```python
from build123d import *

# Parameters (mm, degrees)
CROQUIS1_W                 = 19.8
CROQUIS1_H                 = 11.5
SALIENTE_EXTRUIR1_DEPTH    = 70.5
VACIADO1_T                 = -2
CROQUIS5_W                 = 15.8
CROQUIS5_H                 = 2
SALIENTE_EXTRUIR2_DEPTH    = 2
CROQUIS6_W                 = 19.8
CROQUIS6_H                 = 8
SALIENTE_EXTRUIR4_DEPTH    = 16
SALIENTE_EXTRUIR5_DEPTH    = 19.8
CROQUIS10_R                = 3
CORTAR_EXTRUIR4_DEPTH      = 19.8
CORTAR_EXTRUIR3_DEPTH      = 43.653516854
CORTAR_EXTRUIR3_DEPTH_BACK = 43.653516854
CROQUIS8_R                 = 1
CROQUIS11_W                = 15.8
CROQUIS11_H                = 26
CORTAR_EXTRUIR5_DEPTH      = 2
REDONDEO2_R                = 8
REDONDEO4_R                = 1
REDONDEO5_R                = 1
REDONDEO6_R                = 1
REDONDEO7_R                = 1
REDONDEO8_R                = 1


# Some blends are built 0.0001 mm under size
with BuildPart() as part:
    # Croquis1 → Saliente-Extruir1 (new body)
    with BuildSketch(Plane(origin=(0, 0, 0), x_dir=(0, 1, 0), z_dir=(0, 0, 1))):
        Rectangle(CROQUIS1_W, CROQUIS1_H)
    extrude(amount=SALIENTE_EXTRUIR1_DEPTH)

    # Vaciado1
    vaciado1_openings = [part.faces().sort_by_distance(p)[0] for p in [
        (0, 0, 70.5),
    ]]
    offset(amount=VACIADO1_T, openings=vaciado1_openings, kind=Kind.INTERSECTION)

    # Croquis5 → Saliente-Extruir2 (add)
    with BuildSketch(Plane.YZ.offset(5.75)):
        with Locations((0, 69.5)):
            Rectangle(CROQUIS5_W, CROQUIS5_H)
    extrude(amount=-SALIENTE_EXTRUIR2_DEPTH)

    # Croquis6 → Saliente-Extruir4 (add)
    with BuildSketch(Plane(origin=(-5.75, 0, 0), x_dir=(0, -1, 0), z_dir=(-1, 0, 0))):
        with Locations((0, 29)):
            Rectangle(CROQUIS6_W, CROQUIS6_H)
    extrude(amount=SALIENTE_EXTRUIR4_DEPTH)

    # Croquis9 → Saliente-Extruir5 (add)
    with BuildSketch(Plane.XZ.offset(9.9)):
        Polygon((-5.75, 70.5), (-12.75, 33), (-5.75, 33), align=None)
        Polygon((-5.75, 0), (-12.75, 25), (-5.75, 25), align=None)
    extrude(amount=-SALIENTE_EXTRUIR5_DEPTH)

    # Croquis10 → Cortar-Extruir4 (cut)
    with BuildSketch(Plane.XZ.offset(9.9)):
        with Locations(Location((-16.745253682, 29, 0), (0, 0, 270))):
            Circle(CROQUIS10_R)
    extrude(amount=-CORTAR_EXTRUIR4_DEPTH, mode=Mode.SUBTRACT)

    # Croquis8 → Cortar-Extruir3 (cut, two sides: drawn at the far end of the back side and taken through both)
    with BuildSketch(Plane(origin=(-4, 0, 33), x_dir=(1, 0, 0), z_dir=(0, 0, 1)).offset(-CORTAR_EXTRUIR3_DEPTH_BACK)):
        with Locations((-12.75, 5.1)):
            Circle(CROQUIS8_R)
        with Locations((-12.75, -4.9)):
            Circle(CROQUIS8_R)
    extrude(amount=CORTAR_EXTRUIR3_DEPTH + CORTAR_EXTRUIR3_DEPTH_BACK, mode=Mode.SUBTRACT)

    # Croquis11 → Cortar-Extruir5 (cut)
    with BuildSketch(Plane.YZ.offset(5.75)):
        with Locations((0, 15)):
            Rectangle(CROQUIS11_W, CROQUIS11_H)
    extrude(amount=-CORTAR_EXTRUIR5_DEPTH, mode=Mode.SUBTRACT)

    # Redondeo2
    # the kernel refuses this fillet: 8 mm, written as the material it adds along each edge
    with BuildSketch(Plane(origin=(5.75, -7.9, 28), x_dir=(0, 1, 0), z_dir=(-1, 0, 0)), Plane(origin=(5.75, 7.9, 28), x_dir=(0, 0, -1), z_dir=(-1, 0, 0))) as redondeo2_piece_1:
        with BuildLine():
            CenterArc((REDONDEO2_R, REDONDEO2_R), REDONDEO2_R, 180, 90)
            Line((0, REDONDEO2_R), (0, 0))
            Line((0, 0), (REDONDEO2_R, 0))
        make_face()
    extrude(amount=2)

    # Redondeo4
    redondeo4_edges = [part.edges().sort_by_distance(p)[0] for p in [
        (-12.75, 0, 33),
    ]]
    fillet(redondeo4_edges, radius=REDONDEO4_R)

    # Redondeo5
    redondeo5_edges = [part.edges().sort_by_distance(p)[0] for p in [
        (5.75, 0, 70.5),
        (-5.75, 0, 70.5),
    ]]
    fillet(redondeo5_edges, radius=REDONDEO5_R)

    # Redondeo6
    redondeo6_edges = [part.edges().sort_by_distance(p)[0] for p in [
        (-12.941660805, -9.9, 33.230748054),
        (-12.941660805, 9.9, 33.230748054),
        (-9.25, 9.9, 51.75),
        (-9.25, -9.9, 51.75),
        (-0.084696812, 9.9, 70.5),
        (5.75, 9.9, 34.75),
        (5.457106781, 9.9, 70.207106781),
        (-5.558339195, 9.9, 70.269251946),
        (-0.084696812, -9.9, 70.5),
        (5.75, -9.9, 34.75),
        (5.457106781, -9.9, 70.207106781),
        (-5.558339195, -9.9, 70.269251946),
        (-17.665303188, 9.9, 33),
        (-17.665303188, -9.9, 33),
    ]]
    fillet(redondeo6_edges, radius=REDONDEO6_R - 0.0001)  # a hair under: the kernel refuses the full size

    # Redondeo7
    redondeo7_edges = [part.edges().sort_by_distance(p)[0] for p in [
        (-0.49995, 9.9, 0),
        (5.75, 0, 0),
        (-0.49995, -9.9, 0),
        (5.457136071, -9.607136071, 0),
        (5.457136071, 9.607136071, 0),
        (-21.75, 0, 25),
    ]]
    fillet(redondeo7_edges, radius=REDONDEO7_R - 0.0001)  # a hair under: the kernel refuses the full size

    # Redondeo8
    redondeo8_edges = [part.edges().sort_by_distance(p)[0] for p in [
        (-21.75, 9.9, 29),
        (-21.75, 0, 33),
        (-21.75, -9.607136071, 32.707136071),
        (-21.75, 9.607136071, 32.707136071),
        (-21.75, -9.9, 29),
        (-16.75005, -9.9, 25),
        (-21.457136071, -9.9, 25.292863929),
        (-16.75005, 9.9, 25),
        (-21.457136071, 9.9, 25.292863929),
    ]]
    fillet(redondeo8_edges, radius=REDONDEO8_R - 0.0001)  # a hair under: the kernel refuses the full size


solid = part.part
```
Work out the finished part from the listing and answer in its coordinate system (mm). A direction names the side the tool comes from. Coordinates: 2 decimals unless noted, no trailing zeros. Order: outer loops, then holes, each group sorted by start corner. A loop starts at its lowest first (then second) coordinate and runs counter-clockwise, first axis right, second up. Notation, with made-up numbers: (25.5, 60) - (36.5, 60) arc R8 ccw to (36.5, 64) - close; hole circle Ø7 at (32, -2.75). An arc over 180 degrees is marked (long way). Answer as a JSON object with one key per item and string values.
1. Find section D-D on y = 5.1. Determine the outline of the cut face in (x, z).
Output values:
{"outline": "(-21.75, 26) arc R1 ccw to (-20.75, 25) - (-17.75, 25) - (-17.75, 26.17) arc R3 cw to (-17.75, 31.83) - (-17.75, 33) - (-20.75, 33) arc R1 ccw to (-21.75, 32) - close; (-15.75, 25) - (-12.75, 25) - (-5.75, 0) - (4.75, 0) arc R1 ccw to (5.75, 1) - (5.75, 2) - (-3.75, 2) - (-3.75, 70.5) - (-4.92, 70.5) arc R1 ccw to (-5.9, 69.68) - (-12.6, 33.82) arc R1 cw to (-13.58, 33) - (-15.75, 33) - (-15.75, 31.83) arc R3 cw to (-15.75, 26.17) - close; (3.75, 26.08) - (5.75, 26.08) - (5.75, 69.5) arc R1 ccw to (4.75, 70.5) - (3.75, 70.5) - close"}
2. A tool of negligible diameter and unlimited length cuts with its end or side. For faces 4 (the face through (-8.92, 9.6, 51.95)), 5 (the face through (-17, 0, 33)), 6 (the face through (1, 0, 2)), 7 (the face through (-17, 0, 25)), 8 (the face through (4, -1, 70.5)), from which of +Z, -Z, +X, -X, +Y, -Y can it reach the whole face along a straight path? Write none if from no direction.
Output values:
{"face 4": "+Z, -X, +Y", "face 5": "+Z, -X, +Y, -Y", "face 6": "+X", "face 7": "-Z, -X, +Y, -Y", "face 8": "+Z, +X, -X, +Y, -Y"}
3. The mould has two halves that part along Y. Classify faces 1 (the face through (-3, 9.9, 36)), 2 (the face through (-3.75, 0, 36)), 3 (the face through (-3, -9.9, 36)): +Y half, -Y half, draft (parallel to the pull), parting line (faces both ways), or undercut.
Output values:
{"face 1": "+Y half", "face 2": "undercut", "face 3": "-Y half"}
4. Find section C-C on x = 0.5. Determine the outline of the cut face in (y, z).
Output values:
{"outline": "(-9.9, 1) arc R1 ccw to (-8.9, 0) - (8.9, 0) arc R1 ccw to (9.9, 1) - (9.9, 69.5) arc R1 ccw to (8.9, 70.5) - (7.9, 70.5) - (7.9, 2) - (-7.9, 2) - (-7.9, 70.5) - (-8.9, 70.5) arc R1 ccw to (-9.9, 69.5) - close"}
5. Find section A-A on z = 29. Determine the outline of the cut face in (x, y), plus the area to 3 significant figures.
Output values:
{"outline": "(-21.75, -8.9) arc R1 ccw to (-20.75, -9.9) - (-19.75, -9.9) - (-19.75, 9.9) - (-20.75, 9.9) arc R1 ccw to (-21.75, 8.9) - close; (-13.75, -9.9) - (4.75, -9.9) arc R1 ccw to (5.75, -8.9) - (5.75, 8.9) arc R1 ccw to (4.75, 9.9) - (-13.75, 9.9) - close; hole (-3.75, -7.9) - (3.75, -7.9) - (3.75, 7.9) - (-3.75, 7.9) - close", "area": "306 mm²"}
6. Each of these flat-tipped pins is pushed along its axis until it touches: P1, Ø3, axis at y = 3, z = 39.5, coming from the -X side; P2, Ø4, axis at x = -16.5, y = -1, coming from the -Z side; P3, Ø5, axis at y = 4, z = 17, coming from the +X side. Where does it stop, or does it pass through?
Output values:
{"P1": "stops at x = -11.82", "P2": "stops at z = 25", "P3": "stops at x = -3.75"}
7. Find section B-B on y = -6.75. Determine the outline of the cut face in (x, z).
Output values:
{"outline": "(-21.75, 26) arc R1 ccw to (-20.75, 25) - (-12.75, 25) - (-5.75, 0) - (4.75, 0) arc R1 ccw to (5.75, 1) - (5.75, 2) - (-3.75, 2) - (-3.75, 70.5) - (-4.92, 70.5) arc R1 ccw to (-5.9, 69.68) - (-12.6, 33.82) arc R1 cw to (-13.58, 33) - (-20.75, 33) arc R1 ccw to (-21.75, 32) - close; (3.75, 24.13) - (5.75, 24.13) - (5.75, 69.5) arc R1 ccw to (4.75, 70.5) - (3.75, 70.5) - close; hole circle Ø6 at (-16.75, 29)"}
8. Consider line 1 (Y direction, x = 0.75, z = 65.5); line 2 (Y direction, x = -16.75, z = 32.25); line 3 (Y direction, x = -16.75, z = 32.45). Determine where each line is inside the solid, lowest interval first.
Output values:
{"line 1": "y = -9.9 to -7.9, 7.9 to 9.9", "line 2": "y = -9.87 to -5.9, -3.9 to 4.1, 6.1 to 9.87", "line 3": "y = -9.79 to -5.9, -3.9 to 4.1, 6.1 to 9.79"}
